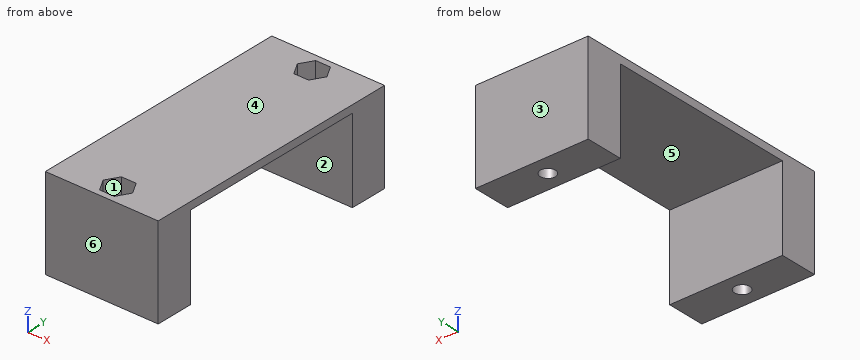
```python
from build123d import *

# Parameters (mm, degrees)
SKETCH2_W           = 30
SKETCH2_H           = 70.4
SKETCH2_R           = 2
BOSS_EXTRUDE1_DEPTH = 2
BOSS_EXTRUDE2_START = -22.26
SKETCH2_2_W         = 30
SKETCH2_2_H         = 10
SKETCH2_2_R         = 2
BOSS_EXTRUDE2_DEPTH = 22.26
CUT_EXTRUDE1_DEPTH  = 14


with BuildPart() as part:
    # Sketch2 → Boss-Extrude1 (new body)
    with BuildSketch(Plane.XY):
        with Locations((-22.5, 3.2)):
            Rectangle(SKETCH2_W, SKETCH2_H)
        with Locations((-22.5, -27)):
            Circle(SKETCH2_R, mode=Mode.SUBTRACT)
        with Locations((-22.5, 33.4)):
            Circle(SKETCH2_R, mode=Mode.SUBTRACT)
    extrude(amount=BOSS_EXTRUDE1_DEPTH)

    # Sketch2<2> → Boss-Extrude2 (add)
    # profile 1 of 2: a face of its own
    with BuildSketch(Plane.XY.offset(BOSS_EXTRUDE2_START)):
        with Locations((-22.5, -27)):
            Rectangle(SKETCH2_2_W, SKETCH2_2_H)
        with Locations(Location((-22.5, -27, 0), (0, 0, 270))):
            Circle(SKETCH2_2_R, mode=Mode.SUBTRACT)
    # profile 2 of 2: a face of its own
    with BuildSketch(Plane.XY.offset(BOSS_EXTRUDE2_START)):
        with Locations((-22.5, 33.4)):
            Rectangle(SKETCH2_2_W, SKETCH2_2_H)
        with Locations(Location((-22.5, 33.4, 0), (0, 0, 270))):
            Circle(SKETCH2_2_R, mode=Mode.SUBTRACT)
    extrude(amount=BOSS_EXTRUDE2_DEPTH)

    # Sketch3 → Cut-Extrude1 (cut)
    with BuildSketch(Plane.XY.offset(2)):
        Polygon((-24.462990915, 30), (-20.537009085, 30), (-18.57401817, 33.4), (-20.537009085, 36.8), (-24.462990915, 36.8), (-26.42598183, 33.4), align=None)
        Polygon((-20.537009085, -30.4), (-18.57401817, -27), (-20.537009085, -23.6), (-24.462990915, -23.6), (-26.42598183, -27), (-24.462990915, -30.4), align=None)
    extrude(amount=-CUT_EXTRUDE1_DEPTH, mode=Mode.SUBTRACT)


solid = part.part
```
Source: CAD feature listing. Evaluate the final solid. Frame: model axes, mm. Face numbers are marked on the shaded views. A direction names the side the tool comes from. Coordinates: 2 decimals unless noted, no trailing zeros. Write each loop counter-clockwise with the first axis right and the second up, starting at its lowest first coordinate (ties: lowest second). Pieces come first, ordered by that corner, then holes. Notation, with made-up numbers: (36.5, 33.5) -> (82.5, 33.5) arc R19 cw to (82.5, 37.5) -> close; hole circle Ø10 at (15.5, 69). An arc over 180 degrees is marked (long way). Return JSON: item names as keys, results as strings. Group by question number.
1) Section query A-A, the plane z = -18.5. Return loops of the section in (x, y).
2) Set-up query: the marked faces 1, 2 and 3. Return all of +Z, -Z, +X, -X, +Y, -Y with unobstructed straight access to the full face (end or side cutting, diameter ignored); none if empty.
3) Section query B-B, the plane x = -22.5. Return loops of the section in (y, z), plus the area to 3 significant figures.
4) Section query D-D, the plane x = -34.5. Return loops of the section in (y, z), plus the area to 3 significant figures.
5) Mould query, pull axis Y, two halves, no side actions, for the marked faces 4, 5 and 6. Classes: +Y half, -Y half, draft (parallel to the pull), parting line (faces both ways), or undercut.
6) Section query C-C, the plane z = -10.5. Return loops of the section in (x, y).
7) Ray query, line 1 along Y through (x, z) = (-23.25, 0.25); line 2 along Y through (x, z) = (-23.5, -11); line 3 along X through (y, z) = (-27, -14.5). Return the intervals inside material, ascending.
8) Contact query for flat-ended pins moving along their axis: P1, Ø1, axis at x = -33.5, y = -19, coming from the -Z side; P2, Ø8, axis at y = -19, z = -2.5, coming from the -X side; P3, Ø2.5, axis at x = -22.5, y = -27, coming from the -Z side; P4, Ø3.5, axis at x = -24, y = -27, coming from the +Z side. Output: stop coordinate, or through.
From the geometry:
{
 "1": {"outline": "(-37.5, -32) -> (-7.5, -32) -> (-7.5, -22) -> (-37.5, -22) -> close; (-37.5, 28.4) -> (-7.5, 28.4) -> (-7.5, 38.4) -> (-37.5, 38.4) -> close; hole circle Ø4 at (-22.5, -27); hole circle Ø4 at (-22.5, 33.4)"},
 "2": {"face 1": "+Z", "face 2": "-Z, +X, -X", "face 3": "+Z, -Z, +X, -X, +Y"},
 "3": {"outline": "(-32, -22.26) -> (-29, -22.26) -> (-29, -12) -> (-30.4, -12) -> (-30.4, 2) -> (-32, 2) -> close; (-25, -22.26) -> (-22, -22.26) -> (-22, 0) -> (28.4, 0) -> (28.4, -22.26) -> (31.4, -22.26) -> (31.4, -12) -> (30, -12) -> (30, 2) -> (-23.6, 2) -> (-23.6, -12) -> (-25, -12) -> close; (35.4, -22.26) -> (38.4, -22.26) -> (38.4, 2) -> (36.8, 2) -> (36.8, -12) -> (35.4, -12) -> close", "area": "314 mm²"},
 "4": {"outline": "(-32, -22.26) -> (-22, -22.26) -> (-22, 0) -> (28.4, 0) -> (28.4, -22.26) -> (38.4, -22.26) -> (38.4, 2) -> (-32, 2) -> close", "area": "586 mm²"},
 "5": {"face 4": "draft", "face 5": "undercut", "face 6": "-Y half"},
 "6": {"outline": "(-37.5, -32) -> (-7.5, -32) -> (-7.5, -22) -> (-37.5, -22) -> close; (-37.5, 28.4) -> (-7.5, 28.4) -> (-7.5, 38.4) -> (-37.5, 38.4) -> close; hole (-26.43, -27) -> (-24.46, -30.4) -> (-20.54, -30.4) -> (-18.57, -27) -> (-20.54, -23.6) -> (-24.46, -23.6) -> close; hole (-26.43, 33.4) -> (-24.46, 30) -> (-20.54, 30) -> (-18.57, 33.4) -> (-20.54, 36.8) -> (-24.46, 36.8) -> close"},
 "7": {"line 1": "-32 to -30.4, -23.6 to 30, 36.8 to 38.4", "line 2": "-32 to -30.4, -23.6 to -22, 28.4 to 30, 36.8 to 38.4", "line 3": "-37.5 to -24.5, -20.5 to -7.5"},
 "8": {"P1": "z = 0", "P2": "x = -37.5", "P3": "through", "P4": "z = -12"}
}
